Autodesk Inventor part; units mm, degrees
ref_plane "YZ Plane" through (0, 0, 0) normal (1, 0, 0) x (0, 1, 0)
ref_plane "XZ Plane" through (0, 0, 0) normal (0, 1, 0) x (-1, 0, 0)
ref_plane "XY Plane" through (0, 0, 0) normal (0, 0, 1) x (1, 0, 0)
sketch "Sketch1" plane through (0, 0, 0) normal (0, 1, 0) x (-1, 0, 0)
  line L0 (0, 0) -> (130.175, 0)
  line L1 (130.175, 0) -> (130.175, -69.85)
  line L2 (130.175, -69.85) -> (0, -69.85)
  line L3 (0, -69.85) -> (0, 0)
  dimension "d0" = 130.175
  dimension "d1" = 69.85
extrude "Extrusion1" add sketch "Sketch1" along normal blind 44.45
sketch "Sketch2" plane through (0, 44.45, 0) normal (0, 1, 0) x (1, 0, 0)
  line L0 (0, 0) -> (0, 69.85)
  line L1 (0, 0) -> (0, 34.925)
  line L2 (0, 34.925) -> (-130.175, 34.925)
  line L3 (-130.175, 69.85) -> (-130.175, 0)
  line L4 (-130.175, 34.925) -> (0, 34.925)
  line L5 (0, 34.925) -> (0, 26.9875)
  line L6 (0, 26.9875) -> (-130.175, 26.9875)
  line L7 (-130.175, 26.9875) -> (-130.175, 34.925)
  line L8 (0, 26.9875) -> (-25.3296, 26.9875)
  line L9 (-25.3296, 26.9875) -> (-25.3296, 42.8625)
  line L10 (-25.3296, 42.8625) -> (0, 42.8625)
  line L11 (0, 42.8625) -> (0, 26.9875)
  line L12 (0, 26.9875) -> (-130.175, 26.9875)
  line L13 (-130.175, 26.9875) -> (-130.175, 42.8625)
  line L14 (-130.175, 42.8625) -> (0, 42.8625)
  line L15 (0, 42.8625) -> (0, 26.9875)
  dimension "d4" = 7.9375
  dimension "d5" = 15.875
extrude "Extrusion2" cut sketch "Sketch2" against normal blind 19.05
chamfer "Chamfer1" distance 25.4 angle 45 2 edges at (0, 44.45, -13.4937) (-130.175, 44.45, -13.4938)
chamfer "Chamfer2" distance 19.05 angle 45 2 edges at (-65.0875, 44.45, 0) (-65.0875, 44.45, -69.85)
properties part number "Block" material "Steel, Mild"
The model under review builds one solid part; all positions refer to its coordinate system, in mm. A direction names the side the tool comes from. Give positions to 0.01 mm unless a question says otherwise; leave off trailing zeros. Write each loop counter-clockwise with the first axis right and the second up, starting at its lowest first coordinate (ties: lowest second). Pieces come first, ordered by that corner, then holes.
(1) Consider section C-C, the plane z = -40.5. Give the boundary of the cut face in (x, y) (3 decimals).
(2) Consider section D-D, the plane x = -58. Give the boundary of the cut face in (y, z).
(3) Consider section B-B, the plane x = -23. Give the boundary of the cut face in (y, z).
(4) For P1, Ø17.5, axis at x = -83, z = -37, coming from the +Y side; P2, Ø9.5, axis at x = -83.5, y = 37.5, coming from the -Z side; P3, Ø12, axis at x = -70.5, y = 32.5, coming from the -Z side; P4, Ø1.5, axis at x = -33.5, z = -7, coming from the +Y side, all flat-tipped, find the tip position at first contact; note any pin that passes through.
(5) The part is to be moulded in two halves that separate along Z. For faces 1 (the flat face through (-64, 35, -26.988)), 2 (the flat face through (-10.06, 29.11, -26.67)), 3 (the flat face through (-64, 13, 0)), say which applies: released by +Z, released by -Z, zero draft, split by the parting line, or undercut.
(6) Tool access review of faces 4 (the flat face through (-64.27, 35.06, -60.19)), 5 (the flat face through (-66, 35, -42.862)): name each direction out of +Z, -Z, +X, -X, +Y, -Y from which nothing blocks a thin tool from reaching the whole face with its end or side.
(7) To check wall thickness, follow L1, parallel to Z at x = -60.5, y = 30; L2, parallel to Z at x = -65, y = 41.5; L3, parallel to Y at x = -44, z = -17.5. State the ranges of each line that lie inside material, in increasing order.
Returned:
1. outline: (-130.175, 0) - (0, 0) - (0, 19.05) - (-6.35, 25.4) - (-123.825, 25.4) - (-130.175, 19.05) - close
2. outline: (0, -69.85) - (25.4, -69.85) - (44.45, -50.8) - (44.45, -42.86) - (25.4, -42.86) - (25.4, -26.99) - (44.45, -26.99) - (44.45, -19.05) - (25.4, 0) - (0, 0) - close
3. outline: (0, -69.85) - (25.4, -69.85) - (42.05, -53.2) - (42.05, -42.86) - (25.4, -42.86) - (25.4, -26.99) - (42.05, -26.99) - (42.05, -16.65) - (25.4, 0) - (0, 0) - close
4. P1: stops at y = 44.45
4. P2: stops at z = -62.5
4. P3: stops at z = -68.75
4. P4: stops at y = 33.15
5. face 1: undercut
5. face 2: zero draft
5. face 3: released by +Z
6. face 4: -Z, +X, -X, +Y
6. face 5: +X, -X, +Y
7. L1: z = -65.25 to -42.86, -26.99 to -4.6
7. L2: z = -53.75 to -42.86, -26.99 to -16.1
7. L3: y = 0 to 42.9
